Can you work these out from the model? Positions are in its coordinate system, mm. Face numbers are marked on the shaded views. A direction names the side the tool comes from. Give positions to 0.01 mm unless a question says otherwise; leave off trailing zeros. Loops run counter-clockwise (first coordinate to the right, second up) from the corner with the lowest first, then second, coordinate; pieces in that order, holes last. Notation, with made-up numbers: (-16, 27) - (-10, 27) arc R12 ccw to (-10, 46) - close; hole circle Ø6 at (32, 29). An arc over 180 degrees is marked (long way). Write item = value, one per line.
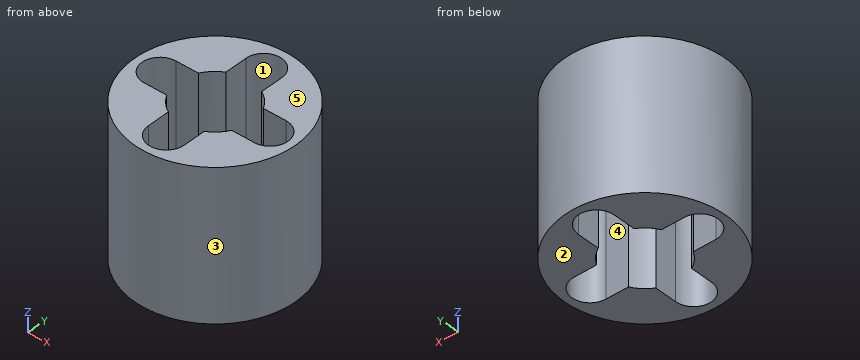
from build123d import *

# Parameters (mm, degrees)
ESQUISSE1_R        = 3.25
BOSS_EXTRU_1_DEPTH = 6


with BuildPart() as part:
    # Esquisse1 → Boss.-Extru.1 (new body)
    with BuildSketch(Plane.XY):
        Circle(ESQUISSE1_R)
        with BuildLine():
            Line((2.225, -0.725), (1.313154599, -0.725))
            ThreePointArc((1.313154599, -0.725), (1.060660172, -1.060660172), (0.725, -1.313154599))
            Line((0.725, -1.313154599), (0.725, -2.225))
            ThreePointArc((0.725, -2.225), (0, -2.95), (-0.725, -2.225))
            Line((-0.725, -2.225), (-0.725, -1.313154599))
            ThreePointArc((-0.725, -1.313154599), (-1.060660172, -1.060660172), (-1.313154599, -0.725))
            Line((-1.313154599, -0.725), (-2.225, -0.725))
            ThreePointArc((-2.225, -0.725), (-2.95, 0), (-2.225, 0.725))
            Line((-2.225, 0.725), (-1.313154599, 0.725))
            ThreePointArc((-1.313154599, 0.725), (-1.060660172, 1.060660172), (-0.725, 1.313154599))
            Line((-0.725, 1.313154599), (-0.725, 2.225))
            ThreePointArc((-0.725, 2.225), (0, 2.95), (0.725, 2.225))
            Line((0.725, 2.225), (0.725, 1.313154599))
            ThreePointArc((0.725, 1.313154599), (1.060660172, 1.060660172), (1.313154599, 0.725))
            Line((1.313154599, 0.725), (2.225, 0.725))
            ThreePointArc((2.225, 0.725), (2.95, 0), (2.225, -0.725))
        make_face(mode=Mode.SUBTRACT)
    extrude(amount=BOSS_EXTRU_1_DEPTH)


solid = part.part
Q1. We'd pull the mould along X, two halves only. Please class the marked faces 1, 2 and 3: released by +X, released by -X, zero draft, split by the parting line, or undercut.
Output:
face_1 = undercut
face_2 = zero draft
face_3 = split by the parting line
Q2. Imagine slicing it at C-C, the plane z = 1.85. Write out the boundary of the cut face in (x, y) (3 decimals), then the cut area to 3 significant figures.
Output:
outline = circle Ø6.5 at (0, 0); hole (-2.225, -0.725) - (-1.313, -0.725) arc R1.5 ccw to (-0.725, -1.313) - (-0.725, -2.225) arc R0.725 ccw to (0.725, -2.225) - (0.725, -1.313) arc R1.5 ccw to (1.313, -0.725) - (2.225, -0.725) arc R0.725 ccw to (2.225, 0.725) - (1.313, 0.725) arc R1.5 ccw to (0.725, 1.313) - (0.725, 2.225) arc R0.725 ccw to (-0.725, 2.225) - (-0.725, 1.313) arc R1.5 ccw to (-1.313, 0.725) - (-2.225, 0.725) arc R0.725 ccw to start
area = 18.3 mm2
Q3. Which directions (+Z, -Z, +X, -X, +Y, -Y) give clear straight access to the entire face, cutting with the end or side of a thin tool? Please do the marked faces 4 and 5.
Output:
face_4 = +Z, -Z
face_5 = +Z, +X, -X, +Y, -Y
Q4. For pin 1 (1.5 mm diameter, centred on y = 1.5, z = 2, fed in from +X); pin 2 (1.5 mm diameter, centred on y = -2.5, z = 3.5, fed in from +X); pin 3 (1 mm diameter, centred on y = -2, z = 3, fed in from +X), each with a flat end and sliding along its axis, tell me the tip position at first contact or that it passes through.
Output:
pin_1 = 3.16
pin_2 = 2.74
pin_3 = 2.88
Q5. I need wall thicknesses on L1, parallel to Y at x = 0, z = 2.35; L2, parallel to Y at x = -2.5, z = 3.3; L3, parallel to X at y = 0.25, z = 4.45. Which ranges of each line are inside material? Lowest first, please.
Output:
L1 = -3.25 to -2.95, 2.95 to 3.25
L2 = -2.08 to -0.67, 0.67 to 2.08
L3 = -3.24 to -2.91, 2.91 to 3.24
Q6. Imagine slicing it at A-A, the plane x = 0. Write out the boundary of the cut face in (y, z), then the cut area to 3 significant figures.
Output:
outline = (-3.25, 0) - (-2.95, 0) - (-2.95, 6) - (-3.25, 6) - close; (2.95, 0) - (3.25, 0) - (3.25, 6) - (2.95, 6) - close
area = 3.60 mm2
